CAD build for the part. Positions are in the model's coordinates, mm. Face numbers are marked on the shaded views. A direction names the side the tool comes from. Round coordinates to 2 decimals unless told otherwise and drop trailing zeros. Write each loop counter-clockwise with the first axis right and the second up, starting at its lowest first coordinate (ties: lowest second). Pieces come first, ordered by that corner, then holes. Notation, with made-up numbers: (3.25, -9.5) - (46.25, -9.5) arc R16 cw to (46.25, -3.5) - close; hole circle Ø10 at (9.5, 8). An arc over 180 degrees is marked (long way). Use one line per item in the form item = value. Start each with the question number.
Item 1: Band-saw the part on A-A, the plane z = 14.5. Give the number of separate pieces and of enclosed holes in the cut face, and give its area (3 significant figures).
Item 2: Pull direction X, two halves, no side cores. Call the marked faces 3, 4, 5 and 6: +X half, -X half, draft (parallel to the pull), parting line (faces both ways), or undercut.
Item 3: Tool access for the marked faces 1 and 2: list every direction of +Z, -Z, +X, -X, +Y, -Y with a clear straight run to the whole face (end or side of a thin tool).
Item 4: Band-saw the part on B-B, the plane x = 38.5. List the corners of the cut face in (y, z), and give its area (3 significant figures).
Item 5: Band-saw the part on D-D, the plane x = 16. List the corners of the cut face in (y, z).
Item 6: Pin check, flat tips, straight feed: pin 1 (10 mm diameter, centred on y = -12.5, z = 8.5, fed in from -X); pin 2 (2 mm diameter, centred on x = -16.5, z = 30, fed in from +Y); pin 3 (8 mm diameter, centred on y = 0, z = 21, fed in from +X). Stop position of each tip, or through.
Item 7: Drill centre lines: L1, parallel to X at y = 0, z = 17; L2, parallel to Z at x = 26, y = -17; L3, parallel to Y at x = -39.5, z = 12.5. Where is each one in solid material? Low to high.
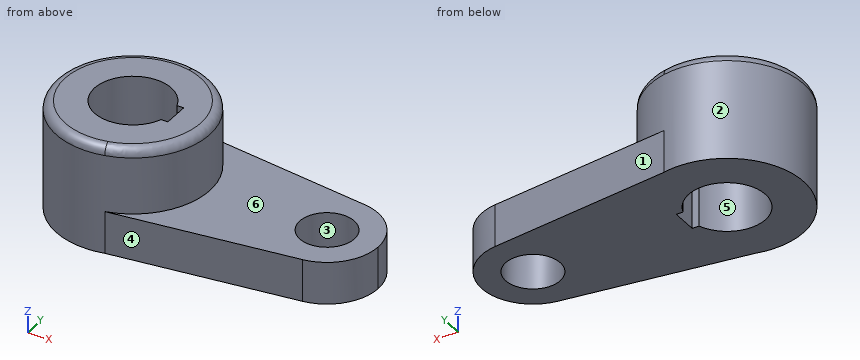
from build123d import *

# Parameters (mm, degrees)
F1_DEPTH = 15.7734
F3_DEPTH = 40.2336
F4_R     = 3.302
F5_R     = 10.16
F6_DEPTH = 40.2346
F8_DEPTH = 40.2346


with BuildPart() as f1:
    # F0 (on Top) → F1 (new body)
    with BuildSketch(Plane.XY):
        with BuildLine():
            ThreePointArc((43.9952853306, -18.8896787473), (55.8448206349, -12.5682112257), (60.5790053739, 0))
            ThreePointArc((60.5790053739, 0), (55.8467902665, 12.565967363), (44.001206343, 18.8889047424))
            ThreePointArc((44.001206343, 18.8889047424), (22.4790056079, 0.0029856939), (43.9952853306, -18.8896787473))
        make_face()
        with BuildLine():
            ThreePointArc((43.9952853306, -18.8896787473), (22.4790056079, 0.0029856939), (44.001206343, 18.8889047424))
            Line((44.001206343, 18.8889047424), (-24.4634996727, 27.8496420043))
            ThreePointArc((-24.4634996727, 27.8496420043), (-8.5077123635, 17.8005889057), (-2.2860042823, 0))
            ThreePointArc((-2.2860042823, 0), (-8.4401964439, -17.7154734872), (-24.2519186042, -27.8001908536))
            Line((-24.2519186042, -27.8001908536), (43.9952853306, -18.8896787473))
        make_face()
        with BuildLine():
            Line((-29.8758121402, 28.5580115107), (-24.4634996727, 27.8496420043))
            ThreePointArc((-24.4634996727, 27.8496420043), (-27.1527028286, 28.3333571136), (-29.8758121402, 28.5580115107))
        make_face()
        with BuildLine():
            ThreePointArc((-2.2860042823, 0), (-8.5077123635, 17.8005889057), (-24.4634996727, 27.8496420043))
            Line((-24.4634996727, 27.8496420043), (-29.8758121402, 28.5580115107))
            ThreePointArc((-29.8758121402, 28.5580115107), (-59.4357622966, 0.1175985837), (-30.110900859, -28.565153069))
            Line((-30.110900859, -28.565153069), (-24.2519186042, -27.8001908536))
            ThreePointArc((-24.2519186042, -27.8001908536), (-8.4401964439, -17.7154734872), (-2.2860042823, 0))
        make_face()
        with BuildLine():
            ThreePointArc((-30.110900859, -28.565153069), (-27.1615843473, -28.3345181209), (-24.2519186042, -27.8001908536))
            Line((-24.2519186042, -27.8001908536), (-30.110900859, -28.565153069))
        make_face()
    extrude(amount=F1_DEPTH)

    # F2 (on Top) → F3 (join)
    with BuildSketch(Plane.XY):
        with BuildLine():
            ThreePointArc((-2.2860042823, 0), (-8.5077123635, 17.8005889057), (-24.4634996727, 27.8496420043))
            ThreePointArc((-24.4634996727, 27.8496420043), (-59.435797755, -0.1086415722), (-24.2519186042, -27.8001908536))
            ThreePointArc((-24.2519186042, -27.8001908536), (-8.4401964439, -17.7154734872), (-2.2860042823, 0))
        make_face()
    extrude(amount=F3_DEPTH)

    # F4
    f4_edges = [f1.edges().sort_by_distance(p)[0] for p in [
        (-37.47009, 27.800191, 40.2336),
    ]]
    fillet(f4_edges, radius=F4_R)

    # F5 (on Top) → F6 (cut, through all)
    with BuildSketch(Plane.XY):
        with Locations((41.5290053739, 0)):
            Circle(F5_R)
    extrude(amount=F6_DEPTH, mode=Mode.SUBTRACT)

    # F7 (on face) → F8 (cut, through all)
    with BuildSketch(Plane.XY.offset(40.2336)):
        with BuildLine():
            ThreePointArc((-17.413239403, -4.826), (-16.7850034837, -2.4492565746), (-16.5735042823, 0))
            ThreePointArc((-16.5735042823, 0), (-16.7850034837, 2.4492565746), (-17.413239403, 4.826))
            ThreePointArc((-17.413239403, 4.826), (-45.1485042823, 0), (-17.413239403, -4.826))
        make_face()
        with BuildLine():
            ThreePointArc((-17.413239403, 4.826), (-16.7850034837, 2.4492565746), (-16.5735042823, 0))
            ThreePointArc((-16.5735042823, 0), (-16.7850034837, -2.4492565746), (-17.413239403, -4.826))
            Line((-17.413239403, -4.826), (-14.8717042823, -4.826))
            Line((-14.8717042823, -4.826), (-14.8717042823, 4.826))
            Line((-14.8717042823, 4.826), (-17.413239403, 4.826))
        make_face()
    extrude(amount=-F8_DEPTH, mode=Mode.SUBTRACT)


solid = f1.part
Determined:
q1.separate_pieces = 1
q1.enclosed_holes = 2
q1.area = 4,340 mm²
q2.face_3 = undercut
q2.face_4 = +X half
q2.face_5 = undercut
q2.face_6 = draft
q3.face_1 = +Z, -Z, +X, +Y
q3.face_2 = +Z
q4.outline = (-19.61, 0) - (-9.7, 0) - (-9.7, 15.77) - (-19.61, 15.77) - close; (9.7, 0) - (19.61, 0) - (19.61, 15.77) - (9.7, 15.77) - close
q4.area = 313 mm²
q5.outline = (-22.54, 0) - (22.55, 0) - (22.55, 15.77) - (-22.54, 15.77) - close
q6.pin_1 = -58.43
q6.pin_2 = 25.26
q6.pin_3 = -2.29
q7.L1 = -59.44 to -45.15, -14.87 to -2.29
q7.L2 = 0 to 15.77
q7.L3 = -27.24 to -11.38, 11.38 to 27.24
